Geometry: final body of the model. Coordinates: model frame, mm. Face numbers are marked on the shaded views. A direction names the side the tool comes from. Round coordinates to 2 decimals unless told otherwise and drop trailing zeros. Write each loop counter-clockwise with the first axis right and the second up, starting at its lowest first coordinate (ties: lowest second). Pieces come first, ordered by that corner, then holes. Notation, with made-up numbers: M 32,-5.75 L 53,-5.75 A21 ccw 53,16.25 Z; hole C 75,-19 d7. An arc over 180 degrees is marked long. Answer as CSV lines item,"result". Start each with the question number.
Q1. First-contact query: pin 1 (4 mm diameter, centred on x = 40.5, y = 10.5, fed in from +Z); pin 2 (5 mm diameter, centred on x = -54.5, y = 11.5, fed in from +Z) (3 decimals); pin 3 (3 mm diameter, centred on y = 18, z = 58.5, fed in from -X). Flat tips, straight axial feed; report the tip coordinate or a pass-through.
Q2. Reachability of the marked faces 5, 6 and 7 from +Z, -Z, +X, -X, +Y, -Y: full face, straight path, thin tool, end or side. Return the list, or none.
Q3. Section query A-A on z = 0. Output: boundary loops of the cut face in (x, y) (3 decimals).
Q4. Section query B-B on x = -28. Output: boundary loops of the cut face in (y, z).
Q5. Section query C-C on z = -39. Output: boundary loops of the cut face in (x, y).
Q6. Ray query, probe 1 along Z at (x, y) = (-57.15, 6.25) (3 decimals); probe 2 along X at (y, z) = (7.75, 0) (3 decimals); probe 3 along Z at (x, y) = (0, 2.25). Return the intervals inside material, ascending.
Q7. Section query D-D on y = 4. Give the number of separate pieces and of enclosed holes in the cut face, and give its area (3 significant figures).
Q8. Mould query, pull axis X, two halves, no side actions, for the marked faces 1, 2, 3 and 4. Classes: pulls with the +X half, pulls with the -X half, needs draft (parallel to the pull), parting line crosses it, or undercut.
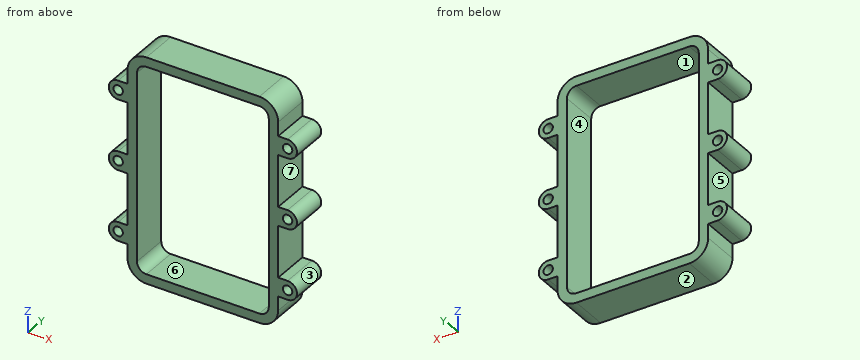
```python
from build123d import *

# Parameters (mm, degrees)
SKETCH1_R           = 3.175
BOSS_EXTRUDE1_DEPTH = 25.4


with BuildPart() as part:
    # Sketch1 → Boss-Extrude1 (new body)
    with BuildSketch(Plane(origin=(0, 0, 0), x_dir=(1, 0, 0), z_dir=(0, 1, 0))):
        with BuildLine():
            Line((0, 76.2), (38.1, 76.2))
            ThreePointArc((38.1, 76.2), (47.080256121, 72.480256121), (50.8, 63.5))
            Line((50.8, 63.5), (50.8, 53.975))
            Line((50.8, 53.975), (57.15, 53.975))
            ThreePointArc((57.15, 53.975), (63.5, 47.625), (57.15, 41.275))
            Line((57.15, 41.275), (50.8, 41.275))
            Line((50.8, 41.275), (50.8, 6.35))
            Line((50.8, 6.35), (57.15, 6.35))
            ThreePointArc((57.15, 6.35), (63.5, 0), (57.15, -6.35))
            Line((57.15, -6.35), (50.8, -6.35))
            Line((50.8, -6.35), (50.8, -41.275))
            Line((50.8, -41.275), (57.15, -41.275))
            ThreePointArc((57.15, -41.275), (63.5, -47.625), (57.15, -53.975))
            Line((57.15, -53.975), (50.8, -53.975))
            Line((50.8, -53.975), (50.8, -63.5))
            ThreePointArc((50.8, -63.5), (47.080256121, -72.480256121), (38.1, -76.2))
            Line((38.1, -76.2), (-4.318973468, -76.2))
            Line((-4.318973468, -76.2), (-38.1, -76.2))
            ThreePointArc((-38.1, -76.2), (-47.080256121, -72.480256121), (-50.8, -63.5))
            Line((-50.8, -63.5), (-50.8, -53.975))
            Line((-50.8, -53.975), (-57.15, -53.975))
            ThreePointArc((-57.15, -53.975), (-63.5, -47.625), (-57.15, -41.275))
            Line((-57.15, -41.275), (-50.8, -41.275))
            Line((-50.8, -41.275), (-50.8, -6.35))
            Line((-50.8, -6.35), (-57.15, -6.35))
            ThreePointArc((-57.15, -6.35), (-63.5, 0), (-57.15, 6.35))
            Line((-57.15, 6.35), (-50.8, 6.35))
            Line((-50.8, 6.35), (-50.8, 41.275))
            Line((-50.8, 41.275), (-57.15, 41.275))
            ThreePointArc((-57.15, 41.275), (-63.5, 47.625), (-57.15, 53.975))
            Line((-57.15, 53.975), (-50.8, 53.975))
            Line((-50.8, 53.975), (-50.8, 63.5))
            ThreePointArc((-50.8, 63.5), (-47.080256121, 72.480256121), (-38.1, 76.2))
            Line((-38.1, 76.2), (0, 76.2))
        make_face()
        with Locations((57.15, 47.625)):
            Circle(SKETCH1_R, mode=Mode.SUBTRACT)
        with Locations((57.15, 0)):
            Circle(SKETCH1_R, mode=Mode.SUBTRACT)
        with Locations((57.15, -47.625)):
            Circle(SKETCH1_R, mode=Mode.SUBTRACT)
        with Locations((-57.15, -47.625)):
            Circle(SKETCH1_R, mode=Mode.SUBTRACT)
        with Locations((-57.15, 47.625)):
            Circle(SKETCH1_R, mode=Mode.SUBTRACT)
        with Locations((-57.15, 0)):
            Circle(SKETCH1_R, mode=Mode.SUBTRACT)
        with BuildLine():
            Line((0, 69.85), (38.1, 69.85))
            ThreePointArc((38.1, 69.85), (42.590128061, 67.990128061), (44.45, 63.5))
            Line((44.45, 63.5), (44.45, -63.5))
            ThreePointArc((44.45, -63.5), (42.590128061, -67.990128061), (38.1, -69.85))
            Line((38.1, -69.85), (-4.318973468, -69.85))
            Line((-4.318973468, -69.85), (-38.1, -69.85))
            ThreePointArc((-38.1, -69.85), (-42.590128061, -67.990128061), (-44.45, -63.5))
            Line((-44.45, -63.5), (-44.45, 63.5))
            ThreePointArc((-44.45, 63.5), (-42.590128061, 67.990128061), (-38.1, 69.85))
            Line((-38.1, 69.85), (0, 69.85))
        make_face(mode=Mode.SUBTRACT)
    extrude(amount=BOSS_EXTRUDE1_DEPTH)


solid = part.part
```
Entries:
1,pin 1,"stops at z = 76.19"
1,pin 2,"stops at z = 53.975"
1,pin 3,"stops at x = -50.8"
2,face 5,"-X, +Y, -Y"
2,face 6,"+Y, -Y"
2,face 7,"+X, +Y, -Y"
3,outline,"M -63.5,0 L -60.325,0 L -60.325,25.4 L -63.5,25.4 Z; M -53.975,0 L -44.45,0 L -44.45,25.4 L -53.975,25.4 Z; M 44.45,0 L 53.975,0 L 53.975,25.4 L 44.45,25.4 Z; M 60.325,0 L 63.5,0 L 63.5,25.4 L 60.325,25.4 Z"
4,outline,"M 0,-76.2 L 25.4,-76.2 L 25.4,-69.85 L 0,-69.85 Z; M 0,69.85 L 25.4,69.85 L 25.4,76.2 L 0,76.2 Z"
5,outline,"M -50.8,0 L -44.45,0 L -44.45,25.4 L -50.8,25.4 Z; M 44.45,0 L 50.8,0 L 50.8,25.4 L 44.45,25.4 Z"
6,probe 1,"z = -53.975 to -50.8, -44.45 to -41.275, -6.35 to -3.175, 3.175 to 6.35, 41.275 to 44.45, 50.8 to 53.975"
6,probe 2,"x = -63.5 to -60.325, -53.975 to -44.45, 44.45 to 53.975, 60.325 to 63.5"
6,probe 3,"z = -76.2 to -69.85, 69.85 to 76.2"
7,separate pieces,"1"
7,enclosed holes,"7"
7,area,"3,630 mm^2"
8,face 1,"undercut"
8,face 2,"needs draft"
8,face 3,"pulls with the +X half"
8,face 4,"undercut"
